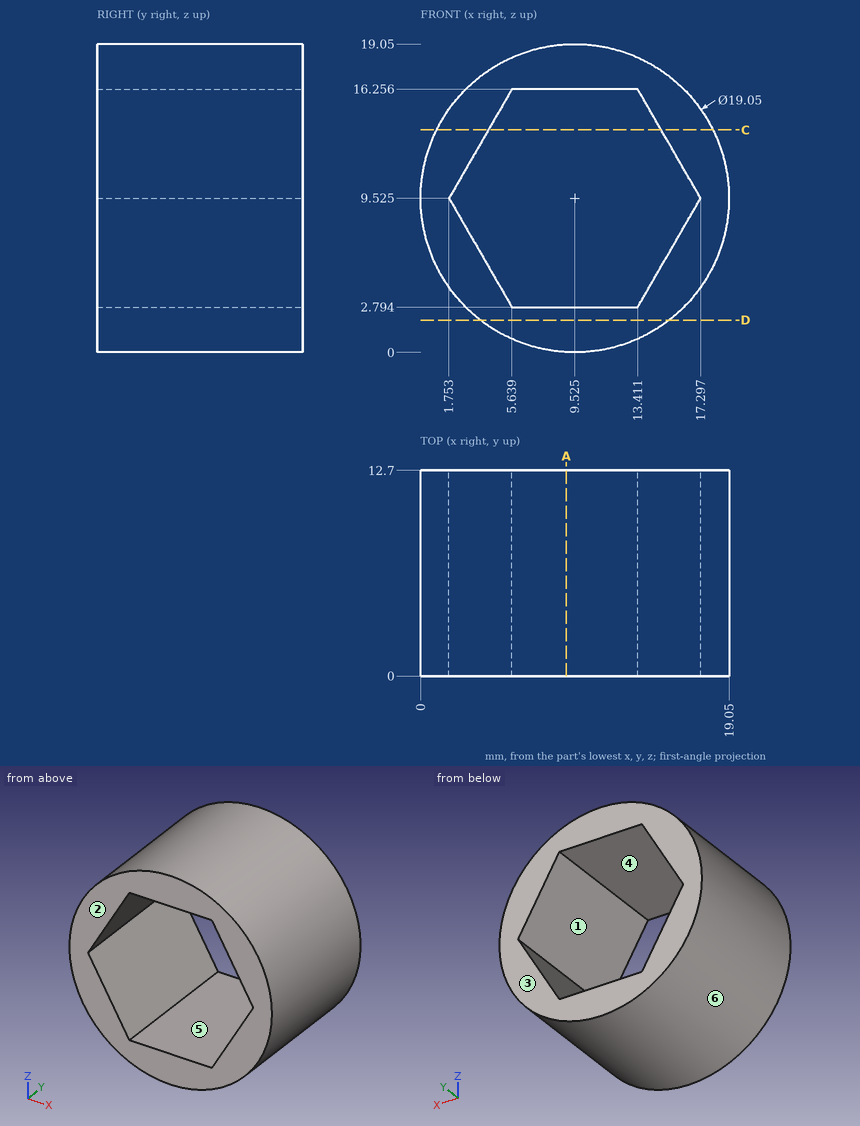
Here's the drawing with two shaded views (mm, measured from the low corner). I have some questions. A direction names the side the tool comes from. Coordinates: 2 decimals unless noted, no trailing zeros. Loops run counter-clockwise (first coordinate to the right, second up) from the corner with the lowest first, then second, coordinate; pieces in that order, holes last. Notation, with made-up numbers: M -35.75,-36 L 3.25,-36 A19 cw 3.25,-29 Z; hole C 43.5,89 d3. An arc over 180 degrees is marked long. Answer as CSV lines item,"result". Start each with the question number.
1. For the marked faces 1 and 2, which set-ups out of +Z, -Z, +X, -X, +Y, -Y let a thin tool reach every point of the face, with its end or its side?
2. Suppose I cut it at D-D, the plane z = 2. List the corners of the cut face in (x, y) for me (1 decimal), plus the area to 3 significant figures.
3. Thinking about a two-plate mould opening in Z: for the marked faces 3, 4, 5 and 6, which applies, +Z half, -Z half, draft (parallel to the pull), parting line (faces both ways), or undercut?
4. Suppose I cut it at C-C, the plane z = 13.75. List the corners of the cut face in (x, y) for me.
5. Suppose I cut it at A-A, the plane x = 9. List the corners of the cut face in (y, z) for me (1 decimal).
6. For pin 1 Ø6 at (y, z) = (11.5, 5.5) entering from +X (1 decimal); pin 2 Ø6 at (y, z) = (7.5, 4.5) entering from -X; pin 3 Ø3 at (x, y) = (6, 9) entering from +Z, each with a flat end and sliding along its axis, tell me the tip position at first contact or that it passes through.
7. If I drill on probe 1 along Z at (x, y) = (9.75, 9.5); probe 2 along Z at (x, y) = (12.75, 1.75) (1 decimal); probe 3 along X at (y, z) = (4.25, 8.75), over which ranges is the centre line in solid material (lowest first)? Write a range as [from, to].
Output:
1,face 1,"+Y, -Y"
1,face 2,"+Z, -Z, +X, -X, -Y"
2,outline,"M 3.7,0 L 15.4,0 L 15.4,12.7 L 3.7,12.7 Z"
2,area,"148 mm^2"
3,face 3,"draft"
3,face 4,"undercut"
3,face 5,"undercut"
3,face 6,"parting line"
4,outline,"M 0.99,0 L 4.19,0 L 4.19,12.7 L 0.99,12.7 Z; M 14.86,0 L 18.06,0 L 18.06,12.7 L 14.86,12.7 Z"
5,outline,"M 0,0 L 12.7,0 L 12.7,2.8 L 0,2.8 Z; M 0,16.3 L 12.7,16.3 L 12.7,19 L 0,19 Z"
6,pin 1,"stops at x = 19"
6,pin 2,"stops at x = 0.22"
6,pin 3,"stops at z = 18.83"
7,probe 1,"z = [0, 2.79], [16.26, 19.05]"
7,probe 2,"z = [0.6, 2.8], [16.3, 18.5]"
7,probe 3,"x = [0.03, 2.2], [16.85, 19.02]"
